Check sheet for the modelled part. Datum: model origin and axes. Units: mm. A direction names the side the tool comes from. Give positions to 0.01 mm unless a question says otherwise; leave off trailing zeros. Order: outer loops, then holes, each group sorted by start corner. A loop starts at its lowest first (then second) coordinate and runs counter-clockwise, first axis right, second up.
```python
from build123d import *

# Parameters (mm, degrees)
BOSS_EXTRUDE1_DEPTH   = 76.2
CUT_EXTRUDE3_DEPTH    = 77.2
CUT_EXTRUDE4_DEPTH    = 77.2
CUT_EXTRUDE5_DEPTH    = 126.785464248
SLANTED_CIRCLE_REACH  = 129.265
SKETCH10_R            = 24.13
BACK_CIRCLE_CUT_REACH = 124.924
SKETCH11_R            = 24.13
FILLET2_R             = 25.4


with BuildPart() as part:
    # Sketch2 → Boss-Extrude1 (new body)
    with BuildSketch(Plane.XY):
        Polygon((0, 203.2), (-31.35093717, 25.4), (-159.146418514, 47.933791374), align=None)
    extrude(amount=-BOSS_EXTRUDE1_DEPTH)

    # Sketch6 → Cut-Extrude3 (cut, through all)
    with BuildSketch(Plane.XY):
        Polygon((-18.598164113, 170.860955123), (-35.036668208, 77.633565709), (-103.699217462, 89.740625707), align=None)
    extrude(amount=-CUT_EXTRUDE3_DEPTH, mode=Mode.SUBTRACT)

    # Sketch8 → Cut-Extrude4 (cut, through all)
    with BuildSketch(Plane.XY):
        Polygon((-124.819846836, 41.881090632), (-116.398812065, 89.639152029), (-159.146418514, 47.933791374), align=None)
    extrude(amount=-CUT_EXTRUDE4_DEPTH, mode=Mode.SUBTRACT)

    # Sketch9 → Cut-Extrude5 (cut, through all)
    with BuildSketch(Plane(origin=(-128.218156228, 22.60832036, 0), x_dir=(0, 0, 1), z_dir=(-0.984807753, 0.173648178, 0))):
        Polygon((-76.2, 19.570083819), (-38.1, 57.670083819), (0, 19.570083819), align=None)
    extrude(amount=-CUT_EXTRUDE5_DEPTH, mode=Mode.SUBTRACT)

    # Sketch10 → Slanted Circle (cut, up to next)
    with BuildSketch(Plane(origin=(-101.569056599, 104.107337538, 0), x_dir=(0.715778778, 0.698327101, 0), z_dir=(-0.698327101, 0.715778778, 0)), mode=Mode.PRIVATE) as slanted_circle_sk1:
        with Locations((40.241649701, 38.1)):
            Circle(SKETCH10_R)
    slanted_circle_tool1 = extrude(slanted_circle_sk1.sketch, amount=-SLANTED_CIRCLE_REACH, mode=Mode.PRIVATE) & part.part
    add(slanted_circle_tool1.solids().sort_by_distance((-72.764938, 132.209172, -38.1))[0], mode=Mode.SUBTRACT)

    # Sketch11 → Back Circle Cut (cut, up to next)
    with BuildSketch(Plane(origin=(-34.749246562, 6.127229728, 0), x_dir=(0, 0, -1), z_dir=(0.984807753, -0.173648178, 0)), mode=Mode.PRIVATE) as back_circle_cut_sk1:
        with Locations((38.1, 136.612935412)):
            Circle(SKETCH11_R)
    back_circle_cut_tool1 = extrude(back_circle_cut_sk1.sketch, amount=-BACK_CIRCLE_CUT_REACH, mode=Mode.PRIVATE) & part.part
    add(back_circle_cut_tool1.solids().sort_by_distance((-11.026659, 140.664708, -38.1))[0], mode=Mode.SUBTRACT)

    # Fillet2
    fillet2_edges = [part.edges().sort_by_distance(p)[0] for p in [
        (-116.398812065, 89.639152029, -38.1),
    ]]
    fillet(fillet2_edges, radius=FILLET2_R)


solid = part.part
```
(1) Cross-section at A-A on y = 54.5. Enter the section's corners in (x, z).
Response values:
outline: (-122.59, -76.2) - (-26.22, -76.2) - (-26.22, -46.65) - (-122.59, -63.39) - close; (-122.59, -12.81) - (-26.22, -29.55) - (-26.22, 0) - (-122.59, 0) - close
(2) Cross-section at D-D on x = -60. Count the separate pieces of the cut face and the enclosed holes in it, then the cut area to 3 significant figures.
Response values:
separate pieces: 3
enclosed holes: 0
area: 2,940 mm2
(3) Cross-section at B-B on z = -24. Enter the section's corners in (x, y).
Response values:
outline: (-120.65, 65.52) - (-27.18, 49.04) - (-14.43, 121.38) - (-26.93, 123.59) - (-35.04, 77.63) - (-103.7, 89.74) - (-80.38, 111.97) - (-86.78, 118.53) - (-110.54, 95.35) arc R25.4 ccw to (-117.82, 81.58) - close; (-58.75, 145.88) - (-52.03, 138.99) - (-18.6, 170.86) - (-20.13, 162.15) - (-7.63, 159.95) - (0, 203.2) - close
(4) Cross-section at C-C on z = -66. Enter the section's corners in (x, y), then the cut area to 3 significant figures.
Response values:
outline: (-123.05, 51.93) - (-29.58, 35.45) - (0, 203.2) - (-110.54, 95.35) arc R25.4 ccw to (-117.82, 81.58) - close; hole (-103.7, 89.74) - (-35.04, 77.63) - (-18.6, 170.86) - close
area: 6,590 mm2
(5) Release check for a two-part mould opening along Z. For faces 4 (the face through (-62, 76, -76.2)), 5 (the face through (-75.385, 52.779, -19.317)), 6 (the face through (-62, 76, 0)), 7 (the face through (-56.045, 148.521, -46.033)) record: released by +Z, released by -Z, zero draft, split by the parting line, or undercut.
Response values:
face 4: released by -Z
face 5: undercut
face 6: released by +Z
face 7: zero draft
(6) Gauge pin test, flat ends, axial feed: pin 1 Ø5 at (x, z) = (-103, -23.5) entering from +Y; pin 2 Ø12 at (x, z) = (-58.5, -68.5) entering from +Y; pin 3 Ø1 at (y, z) = (110, -46.5) entering from +X. Record the tip position at first contact, or that the pin passes through.
Response values:
pin 1: stops at y = 105.15
pin 2: stops at y = 151.98
pin 3: stops at x = -16.35
(7) Material ranges on L1, parallel to Y at x = -57, z = -18.5; L2, parallel to Y at x = -98.5, z = -13.5; L3, parallel to Z at x = -57, y = 139, recorded low to high.
Response values:
L1: y = 48.71 to 81.51, 136.21 to 147.59
L2: y = 50.95 to 88.82, 94.7 to 107.1
L3: z = -76.2 to -56.14, -20.06 to 0
(8) Set-up check for faces 1 (the face through (-68.887, 83.602, -37.567)), 2 (the face through (-75.48, 52.25, -57.42)), 3 (the face through (-86.69, 111.96, -39.16)): record each of +Z, -Z, +X, -X, +Y, -Y from which the full face is reachable in a straight line by a thin tool's end or side.
Response values:
face 1: +Z, -Z
face 2: -X, -Y
face 3: none
